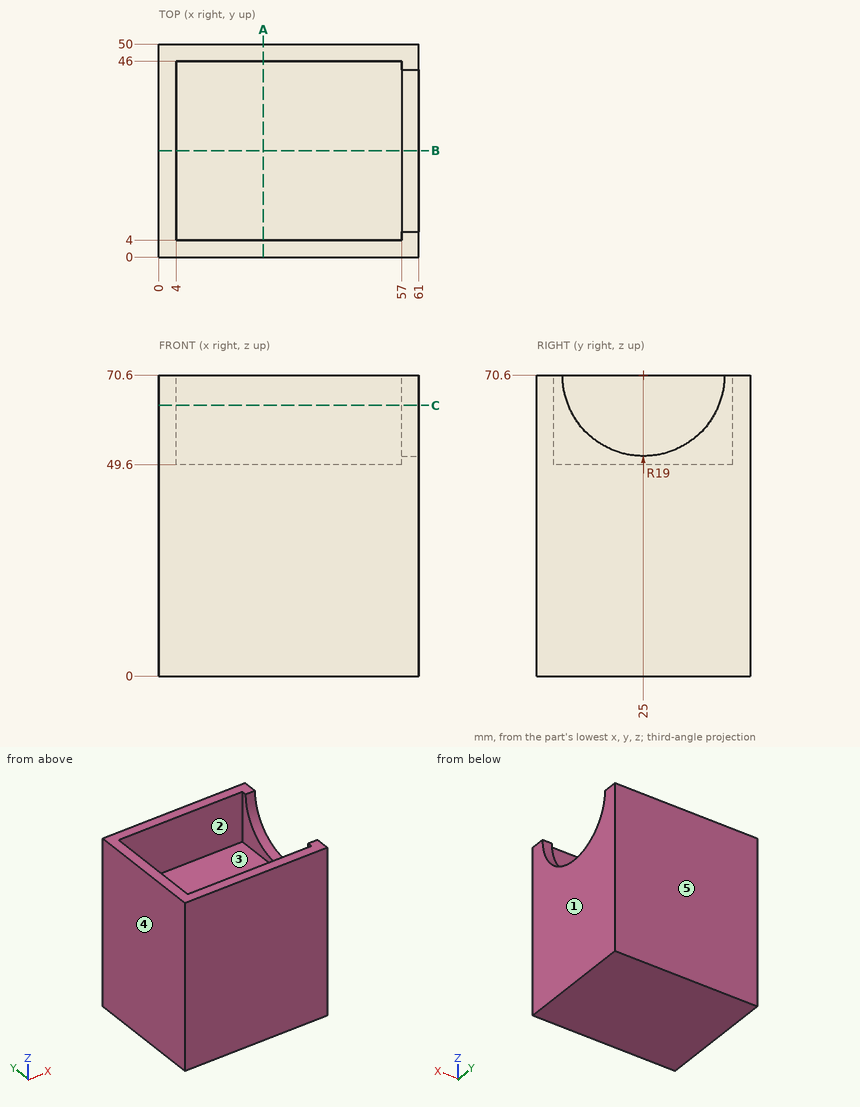
Design review of the part shown in the three views and the two pictorial views. Dimensions are in mm from the part's minimum x, y and z. A direction names the side the tool comes from. Give positions to 0.01 mm unless a question says otherwise; leave off trailing zeros. Loops run counter-clockwise (first coordinate to the right, second up) from the corner with the lowest first, then second, coordinate; pieces in that order, holes last. Notation, with made-up numbers: (79.25, -31.75) -> (128.25, -31.75) arc R12 ccw to (128.25, -17.75) -> close; hole circle Ø4 at (48.5, -23). An arc over 180 degrees is marked (long way). Write each question's results on one line, items separated by ' | '.
Q1. Wall thickness on L1, parallel to X at y = 39.5, z = 57.5; L2, parallel to Y at x = 49.5, z = 58; L3, parallel to Z at x = 43.5, y = 19: over which ranges is each line inside the solid? List them lowest first.
Reply:
L1: x = 0 to 4, 57 to 61 | L2: y = 0 to 4, 46 to 50 | L3: z = 0 to 49.6
Q2. Take a section at A-A, the plane x = 24.5. Write out the cut boundary in (y, z), plus the area to 3 significant figures.
Reply:
outline: (0, 0) -> (50, 0) -> (50, 70.6) -> (46, 70.6) -> (46, 49.6) -> (4, 49.6) -> (4, 70.6) -> (0, 70.6) -> close | area: 2,650 mm²
Q3. The part is to be moulded in two halves that separate along Y. For the marked faces 3, 4 and 5, say which applies: +Y half, -Y half, draft (parallel to the pull), parting line (faces both ways), or undercut.
Reply:
face 3: undercut | face 4: draft | face 5: +Y half
Q4. Machinability: for the marked faces 1 and 2, which of the approach directions +Z, -Z, +X, -X, +Y, -Y give a long, thin tool a straight path to every point of the face, cutting with its end or side? Answer none if there is none.
Reply:
face 1: +Z, -Z, +X, +Y, -Y | face 2: +Z
Q5. Take a section at B-B, the plane y = 25. Write out the cut boundary in (x, z), plus the area to 3 significant figures.
Reply:
outline: (0, 0) -> (61, 0) -> (61, 51.6) -> (57, 51.6) -> (57, 49.6) -> (4, 49.6) -> (4, 70.6) -> (0, 70.6) -> close | area: 3,120 mm²
Q6. Take a section at C-C, the plane z = 63.5. Write out the cut boundary in (x, y).
Reply:
outline: (0, 0) -> (61, 0) -> (61, 7.38) -> (57, 7.38) -> (57, 4) -> (4, 4) -> (4, 46) -> (57, 46) -> (57, 42.62) -> (61, 42.62) -> (61, 50) -> (0, 50) -> close
Q7. For pin 1 Ø10 at (x, y) = (11.5, 22) entering from +Z, flat-tipped, find the tip position at first contact; note if it passes through.
Reply:
pin 1: stops at z = 49.6
